Autodesk Inventor part; units mm, degrees
ref_plane "YZ Plane" through (0, 0, 0) normal (1, 0, 0) x (0, 1, 0)
ref_plane "XZ Plane" through (0, 0, 0) normal (0, 1, 0) x (-1, 0, 0)
ref_plane "XY Plane" through (0, 0, 0) normal (0, 0, 1) x (1, 0, 0)
sketch "Sketch1" plane through (0, 0, 0) normal (0, 0, 1) x (1, 0, 0)
  circle A0 centre (0, 0) radius 37.5
  dimension "d0" = 75
extrude "Extrusion1" add sketch "Sketch1" along normal mid plane 110
sketch "Sketch4" plane through (0, 0, -55) normal (0, 0, -1) x (-1, 0, 0)
  point P0 (0, 0)
  point P1 (0, 0)
hole "Hole1" at (0, 0, -55) direction (0, 0, 1) diameter 26 depth 14 counterbore diameter 30.2 counterbore depth 9
sketch "Sketch5" plane through (0, 0, 55) normal (0, 0, 1) x (1, 0, 0)
  circle A0 centre (0, 0) radius 2.6
  dimension "d22" = 5.2
extrude "Extrusion4" cut sketch "Sketch5" against normal blind 20
properties part number "13042026-11"
CAD build for the part. Positions are in the model's coordinates, mm. A direction names the side the tool comes from. Coordinates: 2 decimals unless noted, no trailing zeros. Order: outer loops, then holes, each group sorted by start corner. A loop starts at its lowest first (then second) coordinate and runs counter-clockwise, first axis right, second up. Notation, with made-up numbers: (-27, -23.75) -> (17, -23.75) arc R14 ccw to (17, 3.25) -> close; hole circle Ø8 at (-36, 64). An arc over 180 degrees is marked (long way). Use one line per item in the form item = value. Start each with the question number.
1) Band-saw the part on D-D on y = -10.5. Give the cut face in (x, z).
2) Drop flat-ended pins along their axis: pin 1 (5 mm diameter, centred on x = -29.5, z = 24.5, fed in from +Y); pin 2 (3 mm diameter, centred on y = 18, z = 10.5, fed in from +X); pin 3 (8 mm diameter, centred on y = 15.5, z = 29.5, fed in from -X). Give the stop position or say it passes through.
3) Tool access for faces 4 (the flat face through (0, 0, 35)), 5 (the flat face through (-12.4, 4.4, -46)), 6 (the flat face through (-1, -8, 55)): list every direction of +Z, -Z, +X, -X, +Y, -Y with a clear straight run to the whole face (end or side of a thin tool).
4) Band-saw the part on A-A on y = 0. Give the cut face in (x, z), then the cut area to 3 significant figures.
5) Band-saw the part on C-C on z = 19.5. Give the cut face in (x, y), then the cut area to 3 significant figures.
6) Drill centre lines: L1, parallel to Y at x = 0, z = 47; L2, parallel to Y at x = 0, z = -51; L3, parallel to Z at x = -0.5, y = 7. Where is each one in solid material? Low to high. Write a range as [from, to].
7) Pull direction Y, two halves, no side cores. Call faces 1 (the flat face through (-1, -16, -55)), 2 (the flat face through (0, 0, -41)), 3 (the cylindrical face through (-4.88, -37.18, -0.77)): +Y half, -Y half, draft (parallel to the pull), parting line (faces both ways), or undercut.
Entries:
q1.outline = (-36, -55) -> (-10.85, -55) -> (-10.85, -46) -> (-7.66, -46) -> (-7.66, -41) -> (7.66, -41) -> (7.66, -46) -> (10.85, -46) -> (10.85, -55) -> (36, -55) -> (36, 55) -> (-36, 55) -> close
q2.pin_1 = 26.02
q2.pin_2 = 33.67
q2.pin_3 = -35.69
q3.face_4 = +Z
q3.face_5 = -Z
q3.face_6 = +Z, +X, -X, +Y, -Y
q4.outline = (-37.5, -55) -> (-15.1, -55) -> (-15.1, -46) -> (-13, -46) -> (-13, -41) -> (13, -41) -> (13, -46) -> (15.1, -46) -> (15.1, -55) -> (37.5, -55) -> (37.5, 55) -> (2.6, 55) -> (2.6, 35) -> (-2.6, 35) -> (-2.6, 55) -> (-37.5, 55) -> close
q4.area = 7,740 mm2
q5.outline = circle Ø75 at (0, 0)
q5.area = 4,420 mm2
q6.L1 = [-37.5, -2.6], [2.6, 37.5]
q6.L2 = [-37.5, -15.1], [15.1, 37.5]
q6.L3 = [-41, 55]
q7.face_1 = draft
q7.face_2 = undercut
q7.face_3 = parting line
